Answer from the drawing. Dimensions are ordinates in mm from the lowest x, y and z of the part. A direction names the side the tool comes from. Coordinates: 2 decimals unless noted, no trailing zeros. Order: outer loops, then holes, each group sorted by start corner. A loop starts at its lowest first (then second) coordinate and runs counter-clockwise, first axis right, second up. Notation, with made-up numbers: M -31.75,-27 L 3.25,-27 A23 ccw 3.25,7 Z; hole C 28.5,23 d9. An arc over 180 degrees is marked long. Use a Markdown table: item, result.
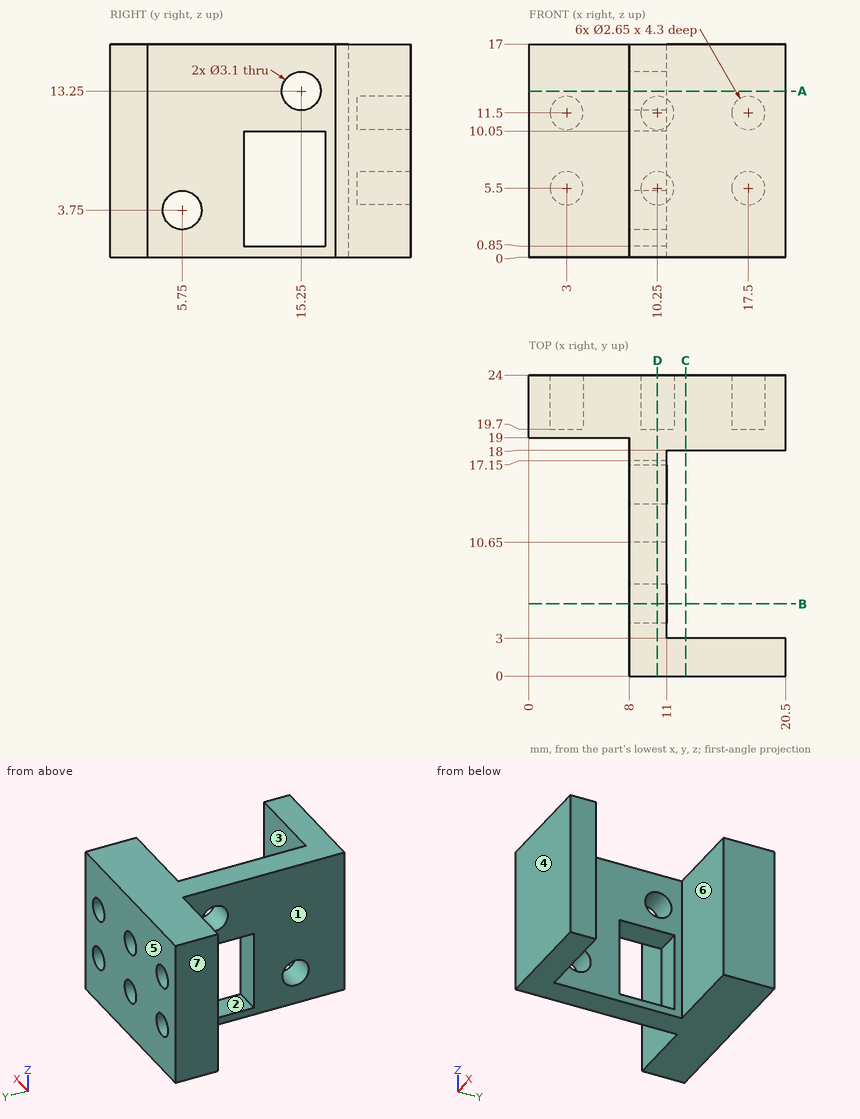
(1) A cutting plane is placed at C-C (x = 12.5). Determine the outline of the cut face in (y, z).
Conclusion:
| item | result |
|---|---|
| outline | M 0,0 L 3,0 L 3,17 L 0,17 Z; M 18,0 L 24,0 L 24,17 L 18,17 Z |
(2) Given P1, Ø4, axis at y = 7.5, z = 2, coming from the +X side; P2, Ø2.5, axis at x = 10.25, z = 5.5, coming from the +Y side; P3, Ø8, axis at y = 9.5, z = 10, coming from the -X side, each flat-ended and moving along its own axis, determine where each tip first touches the part or whether it passes through.
Conclusion:
| item | result |
|---|---|
| P1 | x = 11 |
| P2 | y = 19.7 |
| P3 | x = 8 |
(3) Which of the six approach directions +Z, -Z, +X, -X, +Y, -Y give full straight-line access (tool end or side, diameter ignored) to the marked faces 1, 2 and 3?
Conclusion:
| item | result |
|---|---|
| face 1 | +Z, -Z, -X, -Y |
| face 2 | +X, -X |
| face 3 | +Z, -Z, +X |
(4) A cutting plane is placed at D-D (x = 10.25). Determine the outline of the cut face in (y, z) (3 decimals), then the cut area to 3 significant figures.
Conclusion:
| item | result |
|---|---|
| outline | M 0,0 L 24,0 L 24,4.175 L 19.7,4.175 L 19.7,6.825 L 24,6.825 L 24,10.175 L 19.7,10.175 L 19.7,12.825 L 24,12.825 L 24,17 L 0,17 Z; hole C 5.75,3.75 d3.1; hole M 10.65,0.85 L 17.15,0.85 L 17.15,10.05 L 10.65,10.05 Z; hole C 15.25,13.25 d3.1 |
| area | 310 mm2 |
(5) A cutting plane is placed at A-A (z = 13.25). Determine the outline of the cut face in (x, y), then the cut area to 3 significant figures.
Conclusion:
| item | result |
|---|---|
| outline | M 0,19 L 8,19 L 8,16.8 L 11,16.8 L 11,18 L 20.5,18 L 20.5,24 L 0,24 Z; M 8,0 L 20.5,0 L 20.5,3 L 11,3 L 11,13.7 L 8,13.7 Z |
| area | 188 mm2 |
(6) A cutting plane is placed at B-B (y = 5.75). Determine the outline of the cut face in (x, z).
Conclusion:
| item | result |
|---|---|
| outline | M 8,0 L 11,0 L 11,2.2 L 8,2.2 Z; M 8,5.3 L 11,5.3 L 11,17 L 8,17 Z |
(7) Determine the mould class of the marked faces 4, 5, 6 and 7 for opening direction Y: pulls with the +Y half, pulls with the -Y half, needs draft (parallel to the pull), parting line crosses it, or undercut.
Conclusion:
| item | result |
|---|---|
| face 4 | pulls with the -Y half |
| face 5 | pulls with the +Y half |
| face 6 | undercut |
| face 7 | needs draft |
(8) Straight lines are drawn through the part: L1, parallel to X at y = 22.1, z = 11.5 (3 decimals); L2, parallel to Y at x = 14.25, z = 7.75; L3, parallel to Z at x = 10.25, y = 21.5 (3 decimals). For each, find the intervals that lie inside material, in ascending order.
Conclusion:
| item | result |
|---|---|
| L1 | 0 to 1.675, 4.325 to 8.925, 11.575 to 16.175, 18.825 to 20.5 |
| L2 | 0 to 3, 18 to 24 |
| L3 | 0 to 4.175, 6.825 to 10.175, 12.825 to 17 |
